from build123d import *

# Parameters (mm, degrees)
CROQUIS1_R                 = 47
SALIENTE_EXTRUIR1_DEPTH    = 2
CROQUIS2_W                 = 54
CROQUIS2_H                 = 28
SALIENTE_EXTRUIR4_DEPTH    = 20
CROQUIS3_R                 = 3.5
CROQUIS3_R_2               = 1.5
SALIENTE_EXTRUIR5_DEPTH    = 5
CROQUIS4_R                 = 1.5
SALIENTE_EXTRUIR6_DEPTH    = 4
CROQUIS5_R                 = 1.5
CORTAR_EXTRUIR1_DEPTH      = 4
CROQUIS6_R                 = 5
CORTAR_EXTRUIR2_DEPTH      = 4
CROQUIS7_R                 = 2
CORTAR_EXTRUIR3_DEPTH      = 2
SALIENTE_EXTRUIR7_START    = 50
SALIENTE_EXTRUIR7_DEPTH    = 50
REDONDEO1_R                = 5
REDONDEO2_R                = 5
SALIENTE_EXTRUIR9_DEPTH    = 50
CORTAR_EXTRUIR6_DEPTH      = 128.666518168
CORTAR_EXTRUIR6_DEPTH_BACK = 128.666518168
CROQUIS12_W                = 6
CROQUIS12_H                = 3


# Read off the part's stored shape, not the designer's step: Cortar-Extruir7
with BuildPart() as part:
    # Croquis1 → Saliente-Extruir1 (new body)
    with BuildSketch(Plane(origin=(0, 0, 0), x_dir=(1, 0, 0), z_dir=(0, 1, 0))):
        with Locations(Location((0, 0, 0), (0, 0, 270))):
            Circle(CROQUIS1_R)
    extrude(amount=SALIENTE_EXTRUIR1_DEPTH)

    # Croquis2 → Saliente-Extruir4 (add)
    with BuildSketch(Plane(origin=(0, 2, 0), x_dir=(1, 0, 0), z_dir=(0, 1, 0))):
        with BuildLine():
            Line((29, -5), (-29, -5))
            Line((-29, -5), (-29, -35))
            Line((-29, -35), (-31.368774283, -35))
            ThreePointArc((-31.368774283, -35), (-30.19232893, -36.019762267), (-28.982753492, -37))
            Line((-28.982753492, -37), (28.982753492, -37))
            ThreePointArc((28.982753492, -37), (30.19232893, -36.019762267), (31.368774283, -35))
            Line((31.368774283, -35), (29, -35))
            Line((29, -35), (29, -5))
        make_face()
        with Locations((0, -21)):
            Rectangle(CROQUIS2_W, CROQUIS2_H, mode=Mode.SUBTRACT)
    extrude(amount=SALIENTE_EXTRUIR4_DEPTH)

    # Croquis3 → Saliente-Extruir5 (add)
    # profile 1 of 4: a face of its own
    with BuildSketch(Plane(origin=(0, 2, 0), x_dir=(1, 0, 0), z_dir=(0, 1, 0))):
        with Locations(Location((-26, 31, 0), (0, 0, 270))):
            Circle(CROQUIS3_R)
        with Locations(Location((-26, 31, 0), (0, 0, 270))):
            Circle(CROQUIS3_R_2, mode=Mode.SUBTRACT)
    # profile 2 of 4: a face of its own
    with BuildSketch(Plane(origin=(0, 2, 0), x_dir=(1, 0, 0), z_dir=(0, 1, 0))):
        with Locations(Location((-26, 9, 0), (0, 0, 270))):
            Circle(CROQUIS3_R)
        with Locations(Location((-26, 9, 0), (0, 0, 270))):
            Circle(CROQUIS3_R_2, mode=Mode.SUBTRACT)
    # profile 3 of 4: a face of its own
    with BuildSketch(Plane(origin=(0, 2, 0), x_dir=(1, 0, 0), z_dir=(0, 1, 0))):
        with Locations(Location((26, 9, 0), (0, 0, 270))):
            Circle(CROQUIS3_R)
        with Locations(Location((26, 9, 0), (0, 0, 270))):
            Circle(CROQUIS3_R_2, mode=Mode.SUBTRACT)
    # profile 4 of 4: a face of its own
    with BuildSketch(Plane(origin=(0, 2, 0), x_dir=(1, 0, 0), z_dir=(0, 1, 0))):
        with Locations(Location((26, 31, 0), (0, 0, 270))):
            Circle(CROQUIS3_R)
        with Locations(Location((26, 31, 0), (0, 0, 270))):
            Circle(CROQUIS3_R_2, mode=Mode.SUBTRACT)
    extrude(amount=SALIENTE_EXTRUIR5_DEPTH)

    # Croquis4 → Saliente-Extruir6 (add)
    # profile 1 of 2: a face of its own
    with BuildSketch(Plane(origin=(0, 22, 0), x_dir=(1, 0, 0), z_dir=(0, 1, 0))):
        with BuildLine():
            Line((-29, -17.5), (-31, -17.5))
            ThreePointArc((-31, -17.5), (-34.5, -21), (-31, -24.5))
            Line((-31, -24.5), (-29, -24.5))
            Line((-29, -24.5), (-29, -17.5))
        make_face()
        with Locations(Location((-31, -21, 0), (0, 0, 270))):
            Circle(CROQUIS4_R, mode=Mode.SUBTRACT)
    # profile 2 of 2: a face of its own
    with BuildSketch(Plane(origin=(0, 22, 0), x_dir=(1, 0, 0), z_dir=(0, 1, 0))):
        with BuildLine():
            ThreePointArc((31, -24.5), (34.5, -21), (31, -17.5))
            Line((31, -17.5), (29, -17.5))
            Line((29, -17.5), (29, -24.5))
            Line((29, -24.5), (31, -24.5))
        make_face()
        with Locations(Location((31, -21, 0), (0, 0, 270))):
            Circle(CROQUIS4_R, mode=Mode.SUBTRACT)
    extrude(amount=-SALIENTE_EXTRUIR6_DEPTH)

    # Croquis5 → Cortar-Extruir1 (cut)
    with BuildSketch(Plane(origin=(0, 2, 0), x_dir=(1, 0, 0), z_dir=(0, 1, 0))):
        with Locations(Location((0, 42, 0), (0, 0, 270))):
            Circle(CROQUIS5_R)
        with Locations(Location((0, -42, 0), (0, 0, 270))):
            Circle(CROQUIS5_R)
        with Locations(Location((42, 0, 0), (0, 0, 270))):
            Circle(CROQUIS5_R)
        with Locations(Location((-42, 0, 0), (0, 0, 270))):
            Circle(CROQUIS5_R)
    extrude(amount=-CORTAR_EXTRUIR1_DEPTH, mode=Mode.SUBTRACT)

    # Croquis6 → Cortar-Extruir2 (cut)
    with BuildSketch(Plane(origin=(0, 2, 0), x_dir=(1, 0, 0), z_dir=(0, 1, 0))):
        with Locations(Location((0, 0, 0), (0, 0, 270))):
            Circle(CROQUIS6_R)
    extrude(amount=-CORTAR_EXTRUIR2_DEPTH, mode=Mode.SUBTRACT)

    # Croquis7 → Cortar-Extruir3 (cut)
    with BuildSketch(Plane(origin=(0, 0, 5), x_dir=(-1, 0, 0), z_dir=(0, 0, -1))):
        with Locations((-23, 12)):
            Circle(CROQUIS7_R)
    extrude(amount=-CORTAR_EXTRUIR3_DEPTH, mode=Mode.SUBTRACT)

    # Croquis8 → Saliente-Extruir7 (add)
    with BuildSketch(Plane.XZ.offset(SALIENTE_EXTRUIR7_START)):
        with BuildLine():
            Line((-25.237363199, -36.042689949), (-26.958092508, -38.500146082))
            ThreePointArc((-26.958092508, -38.500146082), (-33.234018716, -33.234018716), (-38.500146082, -26.958092508))
            Line((-38.500146082, -26.958092508), (-36.042689949, -25.237363199))
            ThreePointArc((-36.042689949, -25.237363199), (-31.112698372, -31.112698372), (-25.237363199, -36.042689949))
        make_face()
        with BuildLine():
            Line((25.237363199, 36.042689949), (26.958092508, 38.500146082))
            ThreePointArc((26.958092508, 38.500146082), (33.234018716, 33.234018716), (38.500146082, 26.958092508))
            Line((38.500146082, 26.958092508), (36.042689949, 25.237363199))
            ThreePointArc((36.042689949, 25.237363199), (31.112698372, 31.112698372), (25.237363199, 36.042689949))
        make_face()
    extrude(amount=-SALIENTE_EXTRUIR7_DEPTH)

    # Redondeo1
    redondeo1_edges = [part.edges().sort_by_distance(p)[0] for p in [
        (37.271418015, -50, 26.097727854),
        (26.097727854, -50, 37.271418015),
    ]]
    fillet(redondeo1_edges, radius=REDONDEO1_R)

    # Redondeo2
    redondeo2_edges = [part.edges().sort_by_distance(p)[0] for p in [
        (-37.271418015, -50, -26.097727854),
        (-26.097727854, -50, -37.271418015),
    ]]
    fillet(redondeo2_edges, radius=REDONDEO2_R)


with BuildPart() as body_2:
    # Croquis9 → Saliente-Extruir9 (new body)
    with BuildSketch(Plane.XZ.offset(50)):
        Polygon((34.648232278, 34.648232278), (32.526911935, 36.769552622), (33.941125497, 38.183766184), (38.183766184, 33.941125497), (36.769552622, 32.526911935), align=None)
    extrude(amount=-SALIENTE_EXTRUIR9_DEPTH)


with BuildPart() as cortar_extruir6_tool:
    # Croquis12 → Cortar-Extruir6 (new, two sides: drawn at the far end of the back side and taken through both)
    with BuildSketch(Plane(origin=(36.062445841, 0, 36.062445841), x_dir=(0.7071067811865475, 0, -0.7071067811865477), z_dir=(0.7071067811865477, 0, 0.7071067811865475)).offset(-CORTAR_EXTRUIR6_DEPTH_BACK)):
        with Locations((0, -44.2)):
            Rectangle(CROQUIS12_W, CROQUIS12_H)
    extrude(amount=CORTAR_EXTRUIR6_DEPTH + CORTAR_EXTRUIR6_DEPTH_BACK)


with BuildPart() as part_1:
    add(part.part)

    # Cortar-Extruir6: cut by cortar_extruir6_tool
    add(cortar_extruir6_tool.part, mode=Mode.SUBTRACT)


with BuildPart() as body_2_1:
    add(body_2.part)

    # Cortar-Extruir6: cut by cortar_extruir6_tool
    add(cortar_extruir6_tool.part, mode=Mode.SUBTRACT)


solid = part_1.part
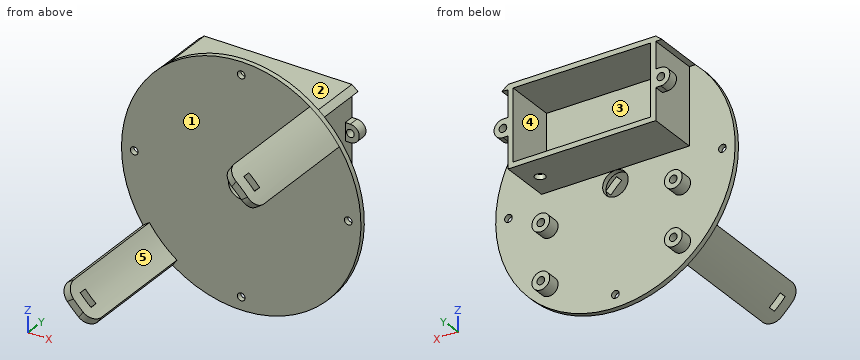
Can you work these out from the model? Positions are in its coordinate system, mm. Face numbers are marked on the shaded views. A direction names the side the tool comes from. Give positions to 0.01 mm unless a question says otherwise; leave off trailing zeros. Write each loop counter-clockwise with the first axis right and the second up, starting at its lowest first coordinate (ties: lowest second). Pieces come first, ordered by that corner, then holes. Notation, with made-up numbers: M 68,47.25 L 109,47.25 A15 cw 109,62.25 Z; hole C -38,42 d5. An arc over 180 degrees is marked long. Answer in a Markdown table with one row per item. Add a question column.
Item 1: Imagine slicing it at A-A, the plane y = -37. Write out the boundary of the cut face in (x, z).
Item 2: On a 3-axis mill with a long thin cutter (end or side, diameter ignored), from which of +Z, -Z, +X, -X, +Y, -Y can I reach the whole of each face in a straight line? I mean the marked faces 4 and 5. Say none if no direction works.
Item 3: For pin 1 Ø4 at (x, z) = (22, -10.5) entering from +Y; pin 2 Ø3.5 at (x, z) = (-42, 0) entering from -Y; pin 3 Ø6 at (y, z) = (-16.5, 22.5) entering from -X, each with a flat end and sliding along its axis, tell me the tip position at first contact or that it passes through.
Item 4: Imagine slicing it at C-C, the plane x = 10.5. Write out the boundary of the cut face in (y, z), plus the area to 3 significant figures.
Item 5: Imagine slicing it at B-B, the plane x = -42. Write out the boundary of the cut face in (y, z), plus the area to 3 significant figures.
Item 6: We'd pull the mould along Z, two halves only. Please class the marked faces 1, 2 and 3: released by +Z, released by -Z, zero draft, split by the parting line, or undercut.
Item 7: Imagine slicing it at D-D, the plane x = -11.5. Write out the boundary of the cut face in (y, z), plus the area to 3 significant figures.
Item 8: Please list where these lines run through material, in increasing order: L1, parallel to X at y = 19.4, z = 21; L2, parallel to X at y = 5, z = -9; L3, parallel to Y at x = -35, z = 29.
Evaluation:
| question | item | result |
|---|---|---|
| 1 | outline | M -38.5,-26.96 A47 ccw -26.96,-38.5 L -25.24,-36.04 A44 cw -36.04,-25.24 Z; M 25.24,36.04 A44 cw 36.04,25.24 L 38.5,26.96 A47 ccw 26.96,38.5 Z |
| 2 | face 4 | +Y |
| 2 | face 5 | +Z, +X, -Y |
| 3 | pin 1 | stops at y = 7 |
| 3 | pin 2 | stops at y = 0 |
| 3 | pin 3 | stops at x = 35.86 |
| 4 | outline | M 0,-45.81 L 2,-45.81 L 2,5 L 22,5 L 22,7 L 2,7 L 2,35 L 22,35 L 22,37 L 2,37 L 2,45.81 L 0,45.81 Z |
| 4 | area | 263 mm² |
| 5 | outline | M 0,-21.1 L 2,-21.1 L 2,-1.5 L 0,-1.5 Z; M 0,1.5 L 2,1.5 L 2,21.1 L 0,21.1 Z |
| 5 | area | 78.4 mm² |
| 6 | face 1 | zero draft |
| 6 | face 2 | released by +Z |
| 6 | face 3 | undercut |
| 7 | outline | M 0,-45.57 L 2,-45.57 L 2,5 L 22,5 L 22,7 L 2,7 L 2,35 L 22,35 L 22,37 L 2,37 L 2,45.57 L 0,45.57 Z |
| 7 | area | 262 mm² |
| 8 | L1 | x = -34.5 to -32.5, -29.5 to -27, 27 to 29.5, 32.5 to 34.5 |
| 8 | L2 | x = -29.5 to -27.5, -24.5 to -22.5, 22.5 to 24.5, 27.5 to 29.5 |
| 8 | L3 | y = 0 to 2 |
